Source: three-view drawing plus pictorial views. Frame: mm from the lowest corner of the part. Give positions to 0.01 mm unless a question says otherwise; leave off trailing zeros. Write each loop counter-clockwise with the first axis right and the second up, starting at its lowest first coordinate (ties: lowest second). Pieces come first, ordered by that corner, then holes.
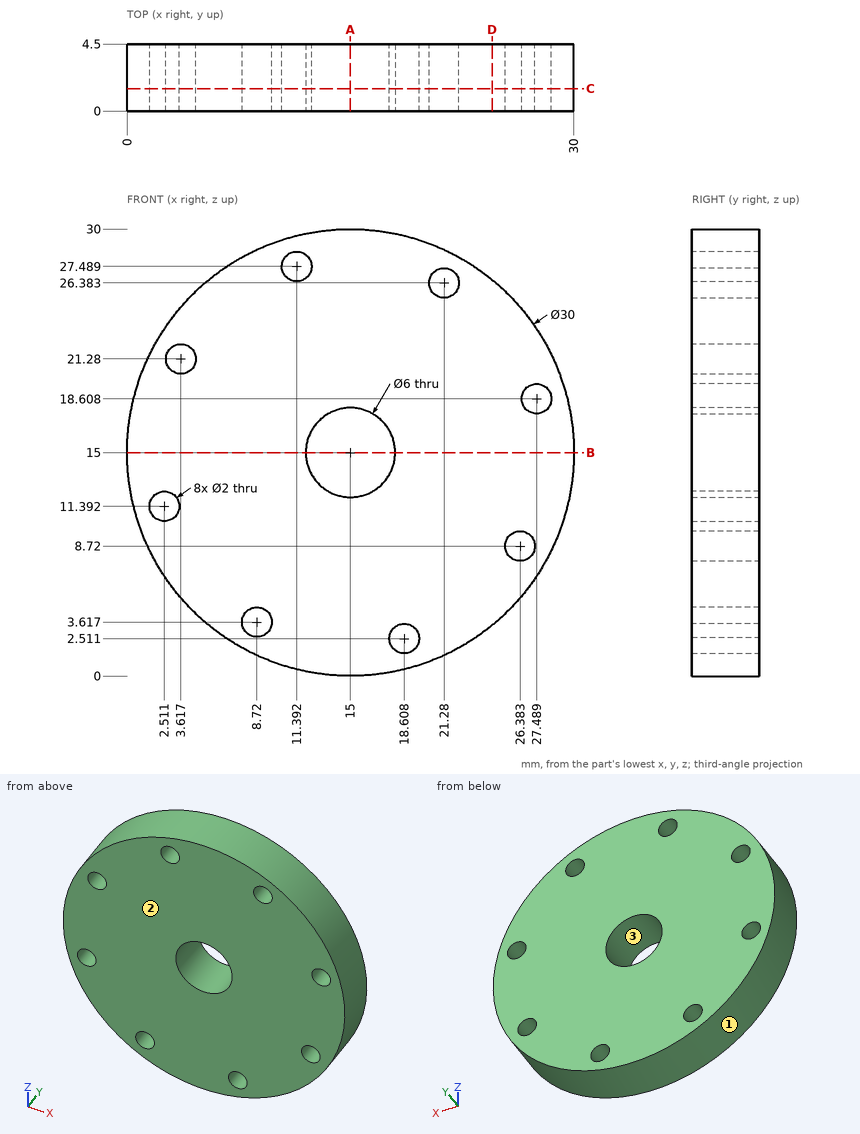
Q1. Ray query, line 1 along X through (y, z) = (1.8, 2.75) (1 decimal); line 2 along Z through (x, y) = (14, 3.55); line 3 along X through (y, z) = (1.25, 3.75). Return the intervals inside material, ascending.
Filled sheet:
line 1: x = 6.3 to 8.2, 9.2 to 17.6, 19.6 to 23.7
line 2: z = 0.03 to 12.17, 17.83 to 29.97
line 3: x = 5.08 to 7.73, 9.71 to 24.92
Q2. Section C-C on y = 1.5. Count the separate pieces of the cut face and the enclosed holes in it.
Filled sheet:
separate pieces: 1
enclosed holes: 9
Q3. Section B-B on z = 15. Output: boundary loops of the cut face in (x, y).
Filled sheet:
outline: (0, 0) - (12, 0) - (12, 4.5) - (0, 4.5) - close; (18, 0) - (30, 0) - (30, 4.5) - (18, 4.5) - close
Q4. Pull-direction query (Z, two-part tool) for the marked faces 1, 2 and 3; classes: released by +Z, released by -Z, zero draft, split by the parting line, or undercut.
Filled sheet:
face 1: split by the parting line
face 2: zero draft
face 3: undercut
Q5. Pin query (flat end, axial travel): P1, Ø1.2, axis at x = 11.39, z = 27.49, coming from the +Y side; P2, Ø1, axis at x = 5.5, y = 3.5, coming from the +Z side; P3, Ø1, axis at x = 21, y = 3, coming from the +Z side (1 decimal); P4, Ø1.5, axis at x = 7.5, y = 2.5, coming from the +Z side (1 decimal). Return the tip coordinate at first contact, or that it passes through.
Filled sheet:
P1: passes through
P2: stops at z = 27
P3: stops at z = 29
P4: stops at z = 28.4
Q6. Section D-D on x = 24.5. Output: boundary loops of the cut face in (y, z).
Filled sheet:
outline: (0, 3.39) - (4.5, 3.39) - (4.5, 26.61) - (0, 26.61) - close
Q7. Section A-A on x = 15. Output: boundary loops of the cut face in (y, z).
Filled sheet:
outline: (0, 0) - (4.5, 0) - (4.5, 12) - (0, 12) - close; (0, 18) - (4.5, 18) - (4.5, 30) - (0, 30) - close
